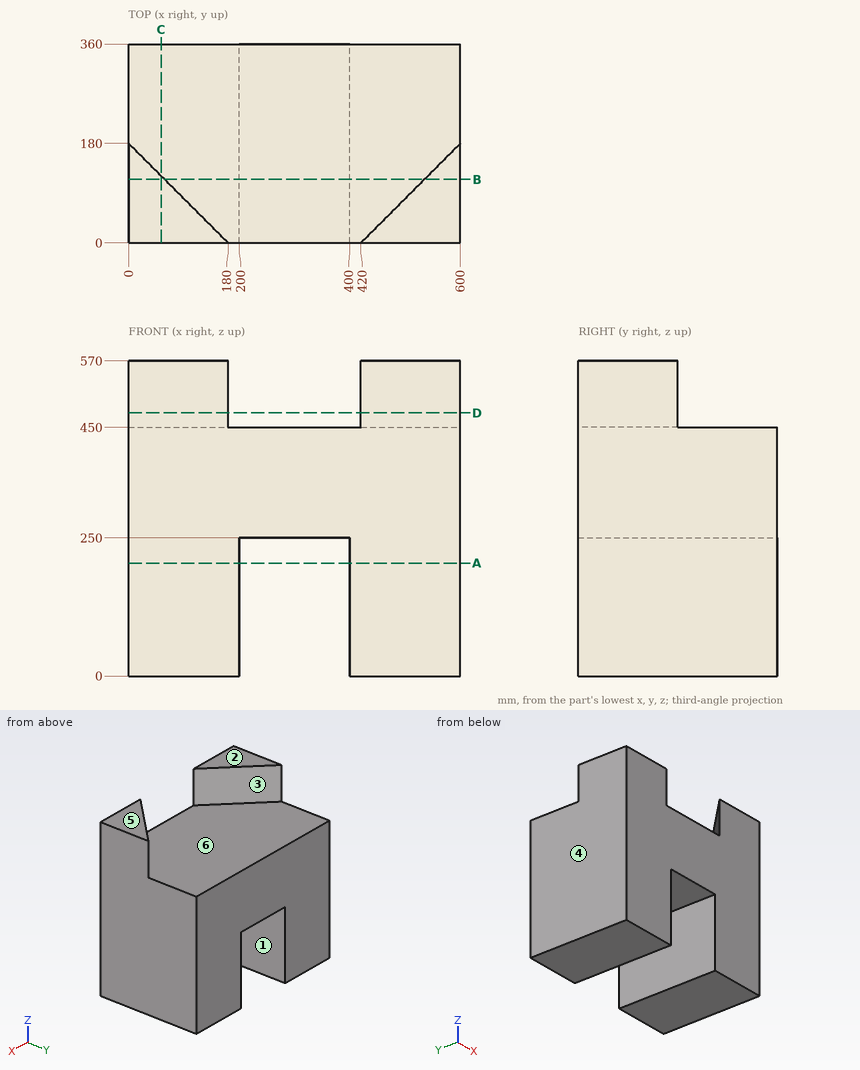
Source: three-view drawing plus pictorial views. Frame: mm from the lowest corner of the part. A direction names the side the tool comes from. Round coordinates to 2 decimals unless told otherwise and drop trailing zeros. Loops run counter-clockwise (first coordinate to the right, second up) from the corner with the lowest first, then second, coordinate; pieces in that order, holes last.
Q1. Section A-A on z = 204. Return loops of the section in (x, y), plus the area to 3 significant figures.
Q2. Pull-direction query (X, two-part tool) for the marked faces 4, 5 and 6; classes: released by +X, released by -X, zero draft, split by the parting line, or undercut.
Q3. Access query for the marked faces 1, 2 and 3. Directions: +Z, -Z, +X, -X, +Y, -Y. A direction counts if a zero-diameter tool reaches every point of the face in a straight line with its end or side. Return the directions, or none.
Q4. Section B-B on y = 115. Return loops of the section in (x, z), plus the area to 3 significant figures.
Q5. Pin query (flat end, axial travel): P1, Ø6, axis at x = 334.5, y = 162.5, coming from the -Z side; P2, Ø4, axis at x = 495.5, y = 86.5, coming from the -Z side; P3, Ø8, axis at x = 163.5, y = 276, coming from the +Z side. Return the tip coordinate at first contact, or that it passes through.
Q6. Material intervals for L1, parallel to X at y = 161, z = 183; L2, parallel to Z at x = 436.5, y = 58; L3, parallel to Z at x = 221.5, y = 85, sorted ascending.
Q7. Section D-D on z = 476. Return loops of the section in (x, y).
Q8. Section C-C on x = 58.5. Return loops of the section in (y, z).
Evaluation:
1. outline: (0, 0) - (200, 0) - (200, 360) - (0, 360) - close; (400, 0) - (600, 0) - (600, 360) - (400, 360) - close
1. area: 144,000 mm2
2. face 4: released by -X
2. face 5: zero draft
2. face 6: undercut
3. face 1: -Z, +Y, -Y
3. face 2: +Z, +X, -X, +Y, -Y
3. face 3: +Z, +Y
4. outline: (0, 0) - (200, 0) - (200, 250) - (400, 250) - (400, 0) - (600, 0) - (600, 570) - (535, 570) - (535, 450) - (65, 450) - (65, 570) - (0, 570) - close
4. area: 236,000 mm2
5. P1: stops at z = 250
5. P2: stops at z = 0
5. P3: stops at z = 450
6. L1: x = 0 to 200, 400 to 600
6. L2: z = 0 to 450
6. L3: z = 250 to 450
7. outline: (0, 0) - (180, 0) - (0, 180) - close; (420, 0) - (600, 0) - (600, 180) - close
8. outline: (0, 0) - (360, 0) - (360, 450) - (121.5, 450) - (121.5, 570) - (0, 570) - close
